Study the drawing (mm; zero at the part's minimum x, y, z) and answer. Coordinates: 2 decimals unless noted, no trailing zeros. Order: outer loops, then holes, each group sorted by start corner. A loop starts at its lowest first (then second) coordinate and runs counter-clockwise, first axis right, second up. Notation, with made-up numbers: M 76,69 L 90,69 A26 cw 90,88 Z; hole C -25,-11.75 d10. An arc over 180 degrees is marked long. Use a Markdown table: item, result. Add a question column.
1) Find section C-C on z = 24.5. Write down the section's boundary in (x, y).
2) Find the intervals of material crossed by probe 1 along Z at (x, y) = (47, 22.5), in increasing order. Write a range as [from, to].
3) Find section A-A on x = 24.5. Write down the section's boundary in (y, z).
4) Find section D-D on y = 34.5. Write down the section's boundary in (x, z), plus the area to 3 significant figures.
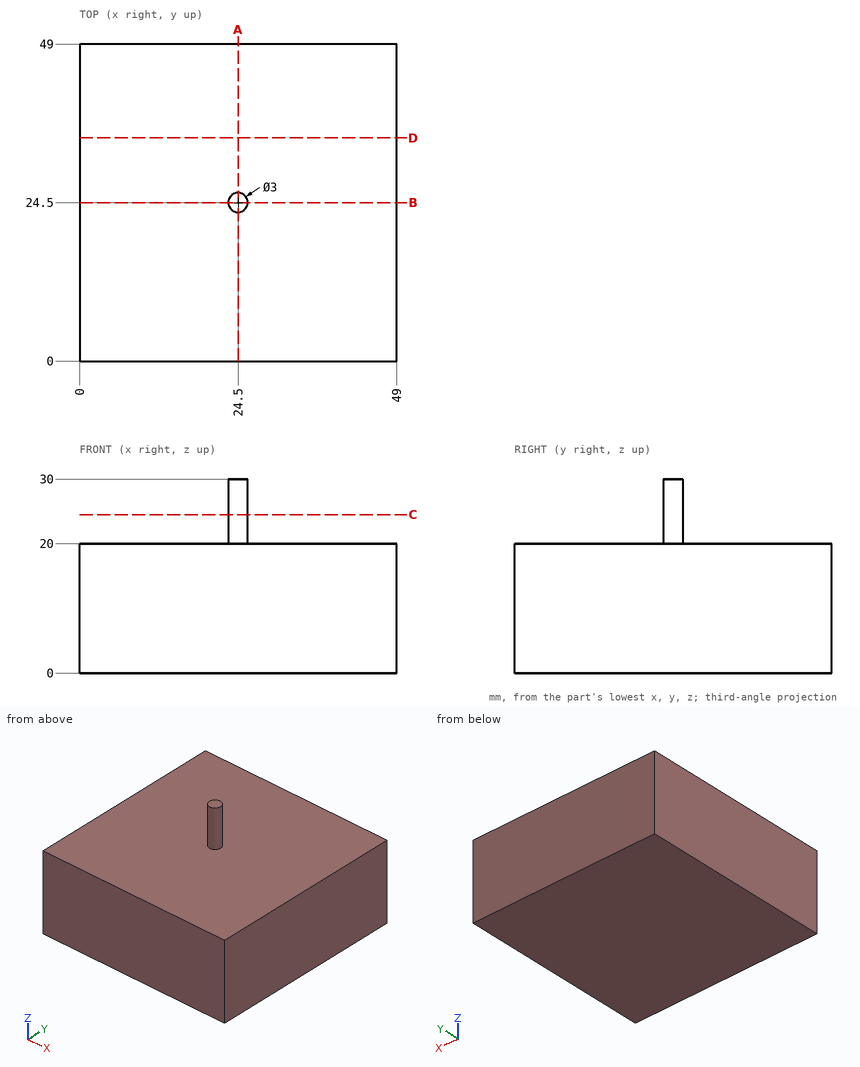
Check result:
| question | item | result |
|---|---|---|
| 1 | outline | C 24.5,24.5 d3 |
| 2 | probe 1 | z = [0, 20] |
| 3 | outline | M 0,0 L 49,0 L 49,20 L 26,20 L 26,30 L 23,30 L 23,20 L 0,20 Z |
| 4 | outline | M 0,0 L 49,0 L 49,20 L 0,20 Z |
| 4 | area | 980 mm2 |
